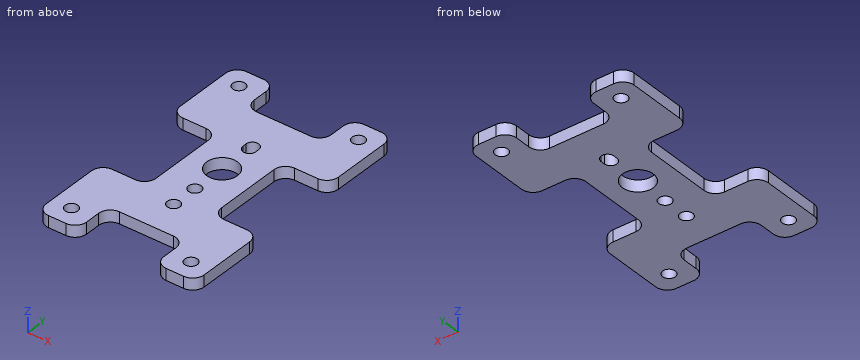
Autodesk Inventor part; units mm, degrees
ref_plane "YZ Plane" through (0, 0, 0) normal (1, 0, 0) x (0, 1, 0)
ref_plane "XZ Plane" through (0, 0, 0) normal (0, 1, 0) x (-1, 0, 0)
ref_plane "XY Plane" through (0, 0, 0) normal (0, 0, 1) x (1, 0, 0)
sketch "Sketch1" plane through (0, 0, 0) normal (0, 0, 1) x (1, 0, 0)
  line L0 (41, 0) -> (41, 65.3) construction
  line L1 (0, 65.3) -> (0, 0) construction
  line L2 (41, 0) -> (41, 21)
  line L3 (0, 21) -> (0, 0)
  line L4 (41, 65.3) -> (41, 44.3)
  line L5 (0, 44.3) -> (0, 65.3)
  line L6 (29, 44.3) -> (29, 21)
  line L7 (12, 21) -> (12, 44.3)
  line L8 (41, 44.3) -> (29, 44.3)
  line L9 (12, 44.3) -> (0, 44.3)
  line L10 (41, 21) -> (29, 21)
  line L11 (12, 21) -> (0, 21)
  line L12 (30.5, 65.3) -> (30.5, 55.3)
  line L13 (30.5, 55.3) -> (10.5, 55.3)
  line L14 (10.5, 55.3) -> (10.5, 65.3)
  line L15 (41, 65.3) -> (30.5, 65.3) construction
  line L16 (10.5, 65.3) -> (0, 65.3) construction
  line L17 (0, 65.3) -> (10.5, 65.3)
  line L18 (30.5, 65.3) -> (41, 65.3)
  line L19 (10.5, 0) -> (10.5, 10)
  line L20 (10.5, 10) -> (30.5, 10)
  line L21 (30.5, 10) -> (30.5, 0)
  line L22 (0, 0) -> (10.5, 0) construction
  line L23 (30.5, 0) -> (41, 0) construction
  line L24 (0, 0) -> (10.5, 0)
  line L25 (30.5, 0) -> (41, 0)
  circle A0 centre (20.5, 35) radius 4
  point P0 (5, 60.3)
  point P1 (36, 60.3)
  point P2 (5, 5)
  point P3 (36, 5)
  point P4 (20.5, 44)
  point P5 (20.5, 26)
  point P6 (20.5, 19)
  point P7 (20.5, 45)
  dimension "d0" = 41
  dimension "d1" = 65.3
  dimension "d2" = 21
  dimension "d3" = 21
  dimension "d4" = 12
  dimension "d5" = 9
  dimension "d6" = 9
  dimension "d7" = 7
  dimension "d8" = 1
  dimension "d9" = 5
  dimension "d11" = 5
  dimension "d12" = 41
  dimension "d13" = 41
  dimension "d14" = 12
  dimension "d15" = 10.5
  dimension "d16" = 10.5
  dimension "d17" = 8
  dimension "d18" = 20.5
  dimension "d19" = 5
  dimension "d20" = 5
extrude "Extrusion1" add sketch "Sketch1" along normal blind 3
sketch "Sketch2" plane through (0, 0, 0) normal (0, 0, 1) x (1, 0, 0)
  line L0 (41, 0) -> (41, 65.3) construction
  line L1 (0, 65.3) -> (0, 0) construction
  line L2 (41, 0) -> (41, 21)
  line L3 (0, 21) -> (0, 0)
  line L4 (41, 65.3) -> (41, 44.3)
  line L5 (0, 44.3) -> (0, 65.3)
  line L6 (29, 44.3) -> (29, 21)
  line L7 (12, 21) -> (12, 44.3)
  line L8 (41, 44.3) -> (29, 44.3)
  line L9 (12, 44.3) -> (0, 44.3)
  line L10 (41, 21) -> (29, 21)
  line L11 (12, 21) -> (0, 21)
  line L12 (30.5, 65.3) -> (30.5, 55.3)
  line L13 (30.5, 55.3) -> (10.5, 55.3)
  line L14 (10.5, 55.3) -> (10.5, 65.3)
  line L15 (41, 65.3) -> (30.5, 65.3) construction
  line L16 (10.5, 65.3) -> (0, 65.3) construction
  line L17 (0, 65.3) -> (10.5, 65.3)
  line L18 (30.5, 65.3) -> (41, 65.3)
  line L19 (10.5, 0) -> (10.5, 10)
  line L20 (10.5, 10) -> (30.5, 10)
  line L21 (30.5, 10) -> (30.5, 0)
  line L22 (0, 0) -> (10.5, 0) construction
  line L23 (30.5, 0) -> (41, 0) construction
  line L24 (0, 0) -> (10.5, 0)
  line L25 (30.5, 0) -> (41, 0)
  circle A0 centre (20.5, 35) radius 4
  point P0 (5, 60.3)
  point P1 (36, 60.3)
  point P2 (5, 5)
  point P3 (36, 5)
  point P4 (20.5, 44)
  point P5 (20.5, 26)
  point P6 (20.5, 19)
  point P7 (20.5, 45)
  dimension "d21" = 41
  dimension "d22" = 65.3
  dimension "d23" = 21
  dimension "d24" = 21
  dimension "d25" = 12
  dimension "d28" = 7
  dimension "d29" = 1
  dimension "d30" = 5
  dimension "d31" = 5
  dimension "d32" = 41
  dimension "d33" = 41
  dimension "d34" = 12
  dimension "d35" = 10.5
  dimension "d36" = 10.5
  dimension "d37" = 8
  dimension "d38" = 20.5
  dimension "d39" = 5
  dimension "d40" = 5
hole "Hole1" at (5, 60.3, 0) at (36, 60.3, 0) at (5, 5, 0) at (36, 5, 0) at (20.5, 44, 0) at (20.5, 26, 0) at (20.5, 19, 0) at (20.5, 45, 0) direction (0, 0, 1) diameter 3.3 end through all
fillet "Fillet1" radius 3 20 edges at (10.5, 65.3, 1.5) (0, 65.3, 1.5) (0, 44.3, 1.5) (12, 44.3, 1.5) (12, 21, 1.5) (0, 21, 1.5) (0, 0, 1.5) (10.5, 0, 1.5) (10.5, 10, 1.5) (30.5, 10, 1.5) (30.5, 0, 1.5) (41, 0, 1.5) (41, 21, 1.5) (29, 21, 1.5) (29, 44.3, 1.5) (41, 44.3, 1.5) (41, 65.3, 1.5) (30.5, 65.3, 1.5) (30.5, 55.3, 1.5) (10.5, 55.3, 1.5)
sketch "Sketch3" plane through (0, 0, 3) normal (0, 0, 1) x (1, 0, 0)
  line L0 (22.15, 45) -> (22.15, 44)
  arc A0 (18.9276, 44.5) -> (22.0724, 44.5) centre (20.5, 44) ccw
  arc A1 (22.0724, 44.5) -> (18.9276, 44.5) centre (20.5, 45) ccw
  line L1 (18.85, 45) -> (18.85, 44)
  point P0 (0, 0)
extrude "Extrusion2" cut sketch "Sketch3" against normal blind 3 contours L0 A0 A1 | A1 A0 L1
sketch "Sketch4" plane through (0, 0, 3) normal (0, 0, 1) x (1, 0, 0)
  circle A0 centre (20.5, 35) radius 4
  circle A1 centre (20.5, 26) radius 1.65
  circle A2 centre (36, 5) radius 1.65
  circle A3 centre (36, 60.3) radius 1.65
  circle A4 centre (5, 60.3) radius 1.65
  circle A5 centre (5, 5) radius 1.65
  line L0 (22.15, 45) -> (22.15, 44)
  arc A6 (18.85, 44) -> (22.15, 44) centre (20.5, 44) ccw
  line L1 (18.85, 44) -> (18.85, 45)
  arc A7 (22.15, 45) -> (18.85, 45) centre (20.5, 45) ccw
  circle A8 centre (20.5, 19) radius 1.65
  arc A9 (33.5, 65.3) -> (30.5, 62.3) centre (33.5, 62.3) ccw
  line L2 (30.5, 62.3) -> (30.5, 58.3)
  arc A10 (27.5, 55.3) -> (30.5, 58.3) centre (27.5, 58.3) ccw
  line L3 (27.5, 55.3) -> (13.5, 55.3)
  arc A11 (10.5, 58.3) -> (13.5, 55.3) centre (13.5, 58.3) ccw
  line L4 (10.5, 58.3) -> (10.5, 62.3)
  arc A12 (10.5, 62.3) -> (7.5, 65.3) centre (7.5, 62.3) ccw
  line L5 (7.5, 65.3) -> (3, 65.3)
  arc A13 (3, 65.3) -> (0, 62.3) centre (3, 62.3) ccw
  line L6 (0, 62.3) -> (0, 47.3)
  arc A14 (0, 47.3) -> (3, 44.3) centre (3, 47.3) ccw
  line L7 (3, 44.3) -> (9, 44.3)
  arc A15 (12, 41.3) -> (9, 44.3) centre (9, 41.3) ccw
  line L8 (12, 41.3) -> (12, 24)
  arc A16 (9, 21) -> (12, 24) centre (9, 24) ccw
  line L9 (9, 21) -> (3, 21)
  arc A17 (3, 21) -> (0, 18) centre (3, 18) ccw
  line L10 (0, 18) -> (0, 3)
  arc A18 (0, 3) -> (3, 0) centre (3, 3) ccw
  line L11 (3, 0) -> (7.5, 0)
  arc A19 (7.5, 0) -> (10.5, 3) centre (7.5, 3) ccw
  line L12 (10.5, 3) -> (10.5, 7)
  arc A20 (13.5, 10) -> (10.5, 7) centre (13.5, 7) ccw
  line L13 (13.5, 10) -> (27.5, 10)
  arc A21 (30.5, 7) -> (27.5, 10) centre (27.5, 7) ccw
  line L14 (30.5, 7) -> (30.5, 3)
  arc A22 (30.5, 3) -> (33.5, 0) centre (33.5, 3) ccw
  line L15 (33.5, 0) -> (38, 0)
  arc A23 (38, 0) -> (41, 3) centre (38, 3) ccw
  line L16 (41, 3) -> (41, 18)
  arc A24 (41, 18) -> (38, 21) centre (38, 18) ccw
  line L17 (38, 21) -> (32, 21)
  arc A25 (29, 24) -> (32, 21) centre (32, 24) ccw
  line L18 (29, 24) -> (29, 41.3)
  arc A26 (32, 44.3) -> (29, 41.3) centre (32, 41.3) ccw
  line L19 (32, 44.3) -> (38, 44.3)
  arc A27 (38, 44.3) -> (41, 47.3) centre (38, 47.3) ccw
  line L20 (41, 47.3) -> (41, 62.3)
  arc A28 (41, 62.3) -> (38, 65.3) centre (38, 62.3) ccw
  line L21 (38, 65.3) -> (33.5, 65.3)
  point P0 (0, 0)
properties part number "TapaInferior"
The listing builds one solid part. Answer for the finished solid, in the listing's coordinates (mm). Coordinates: 2 decimals unless noted, no trailing zeros. Write each loop counter-clockwise with the first axis right and the second up, starting at its lowest first coordinate (ties: lowest second). Pieces come first, ordered by that corner, then holes.
Q1. Find the intervals of material crossed by line 1 along Y through (x, z) = (5, 2); line 2 along Y through (x, z) = (20.5, 1.3); line 3 along X through (y, z) = (5, 2.1), in increasing order.
Returned:
line 1: y = 0 to 3.35, 6.65 to 21, 44.3 to 58.65, 61.95 to 65.3
line 2: y = 10 to 17.35, 20.65 to 24.35, 27.65 to 31, 39 to 42.35, 46.65 to 55.3
line 3: x = 0 to 3.35, 6.65 to 10.5, 30.5 to 34.35, 37.65 to 41
Q2. Section C-C, the plane y = 26 is taken. Write down the section's boundary in (x, z), then the cut area to 3 significant figures.
Returned:
outline: (12, 0) - (18.85, 0) - (18.85, 3) - (12, 3) - close; (22.15, 0) - (29, 0) - (29, 3) - (22.15, 3) - close
area: 41.1 mm2
Q3. Given P1, Ø2.5, axis at x = 5, y = 60.3, coming from the +Z side; P2, Ø1.1, axis at y = 44.5, z = 1.5, coming from the -X side, each flat-ended and moving along its own axis, determine where each tip first touches the part or whether it passes through.
Returned:
P1: passes through
P2: stops at x = 1.02
Q4. Section D-D, the plane z = 1.05 is taken. Give the number of separate pieces and of enclosed holes in the cut face, then the cut area to 3 significant figures.
Returned:
separate pieces: 1
enclosed holes: 8
area: 1,600 mm2
Q5. Section B-B, the plane y = 5 is taken. Write down the section's boundary in (x, z), then the cut area to 3 significant figures.
Returned:
outline: (0, 0) - (3.35, 0) - (3.35, 3) - (0, 3) - close; (6.65, 0) - (10.5, 0) - (10.5, 3) - (6.65, 3) - close; (30.5, 0) - (34.35, 0) - (34.35, 3) - (30.5, 3) - close; (37.65, 0) - (41, 0) - (41, 3) - (37.65, 3) - close
area: 43.2 mm2
Q6. Section A-A, the plane x = 36 is taken. Write down the section's boundary in (y, z), then the cut area to 3 significant figures.
Returned:
outline: (0, 0) - (3.35, 0) - (3.35, 3) - (0, 3) - close; (6.65, 0) - (21, 0) - (21, 3) - (6.65, 3) - close; (44.3, 0) - (58.65, 0) - (58.65, 3) - (44.3, 3) - close; (61.95, 0) - (65.3, 0) - (65.3, 3) - (61.95, 3) - close
area: 106 mm2
